Part model, mm, in its own coordinate system. Round coordinates to 2 decimals unless told otherwise and drop trailing zeros. Loops run counter-clockwise (first coordinate to the right, second up) from the corner with the lowest first, then second, coordinate; pieces in that order, holes last. Notation, with made-up numbers: (79, 8.25) - (111, 8.25) arc R21 ccw to (111, 14.25) - close; hole circle Ø3 at (40.5, -9). An arc over 180 degrees is marked (long way). Put each result on its own line as item: value.
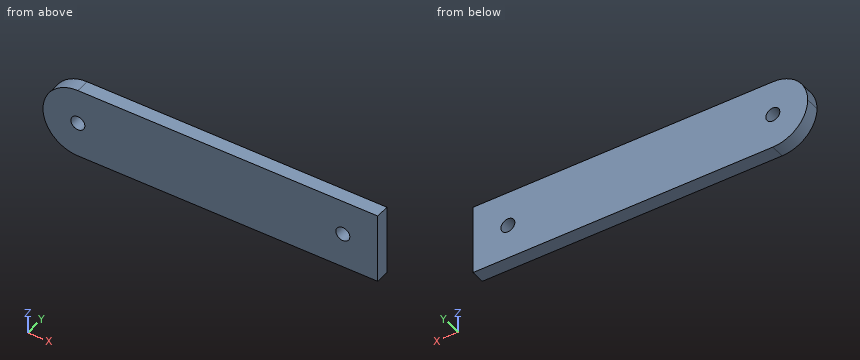
from build123d import *

# Parameters (mm, degrees)
F0_W     = 48
F0_H     = 10
F0_R     = 1
F1_DEPTH = 2
F2_R     = 4.99999


# Not quite as in the source:
# - a fillet or chamfer is up to 0.001 mm smaller than in the source, because OpenCascade refuses the exact size


with BuildPart() as f1:
    # F0 (on Front) → F1 (new body)
    with BuildSketch(Plane.XZ):
        with Locations((24, -5)):
            Rectangle(F0_W, F0_H)
        with Locations((5, -5)):
            Circle(F0_R, mode=Mode.SUBTRACT)
        with Locations((43, -5)):
            Circle(F0_R, mode=Mode.SUBTRACT)
    extrude(amount=F1_DEPTH)

    # F2 (radius 5 in the source; OpenCascade refuses exactly that, so slightly less here)
    f2_edges = [f1.edges().sort_by_distance(p)[0] for p in [
        (0, -1, 0),
        (0, -1, -10),
    ]]
    fillet(f2_edges, radius=F2_R)


solid = f1.part
1. Band-saw the part on C-C (z = -5.5). List the corners of the cut face in (x, y), plus the area to 3 significant figures.
A:
outline: (0.03, -2) - (4.13, -2) - (4.13, 0) - (0.03, 0) - close; (5.87, -2) - (42.13, -2) - (42.13, 0) - (5.87, 0) - close; (43.87, -2) - (48, -2) - (48, 0) - (43.87, 0) - close
area: 89.0 mm²
2. Band-saw the part on D-D (z = -9). List the corners of the cut face in (x, y).
A:
outline: (2, -2) - (48, -2) - (48, 0) - (2, 0) - close
3. Probe line 1 along Z through (x, y) = (43, -0.6); line 2 along X through (y, z) = (-1.05, -5.75); line 3 along X through (y, z) = (-1.45, -5.5). List the from-to ranges inside material, lowest first. Write a range as [from, to].
A:
line 1: z = [-10, -6], [-4, 0]
line 2: x = [0.06, 4.34], [5.66, 42.34], [43.66, 48]
line 3: x = [0.03, 4.13], [5.87, 42.13], [43.87, 48]
4. Band-saw the part on B-B (y = -0.6). Give the number of separate pieces and of enclosed holes in the cut face, plus the area to 3 significant figures.
A:
separate pieces: 1
enclosed holes: 2
area: 463 mm²
5. Band-saw the part on A-A (x = 43). List the corners of the cut face in (y, z), plus the area to 3 significant figures.
A:
outline: (-2, -10) - (0, -10) - (0, -6) - (-2, -6) - close; (-2, -4) - (0, -4) - (0, 0) - (-2, 0) - close
area: 16.0 mm²
